from build123d import *

# Parameters (mm, degrees)
BOSS_EXTRUDE1_DEPTH = 3.03
BOSS_EXTRUDE2_DEPTH = 1
SKETCH3_W           = 1.3
SKETCH3_H           = 3
SKETCH3_W_2         = 1.5
SKETCH3_H_2         = 1.3
BOSS_EXTRUDE3_DEPTH = 5
BOSS_EXTRUDE4_DEPTH = 3
BOSS_EXTRUDE5_DEPTH = 1.5
SKETCH9_W           = 0.5
SKETCH9_H           = 2.5
BOSS_EXTRUDE6_DEPTH = 2
CUT_EXTRUDE1_DEPTH  = 0.5
SKETCH11_W          = 0.25
SKETCH11_H          = 2.5
BOSS_EXTRUDE7_DEPTH = 2
CUT_EXTRUDE2_DEPTH  = 0.25


with BuildPart() as part:
    # Sketch1 → Boss-Extrude1 (new body)
    with BuildSketch(Plane(origin=(0, 0, 0), x_dir=(1, 0, 0), z_dir=(0, 1, 0))):
        with BuildLine():
            Line((-16.7, -3.7), (16.7, -3.7))
            ThreePointArc((16.7, -3.7), (17.407106781, -3.407106781), (17.7, -2.7))
            Line((17.7, -2.7), (17.7, 2.7))
            ThreePointArc((17.7, 2.7), (17.407106781, 3.407106781), (16.7, 3.7))
            Line((16.7, 3.7), (-16.7, 3.7))
            ThreePointArc((-16.7, 3.7), (-17.407106781, 3.407106781), (-17.7, 2.7))
            Line((-17.7, 2.7), (-17.7, -2.7))
            ThreePointArc((-17.7, -2.7), (-17.407106781, -3.407106781), (-16.7, -3.7))
        make_face()
    extrude(amount=BOSS_EXTRUDE1_DEPTH)

    # Sketch2 → Boss-Extrude2 (add)
    with BuildSketch(Plane.XZ):
        with BuildLine():
            Line((16.7, 5.2), (-16.7, 5.2))
            ThreePointArc((-16.7, 5.2), (-18.467766953, 4.467766953), (-19.2, 2.7))
            Line((-19.2, 2.7), (-19.2, -2.7))
            ThreePointArc((-19.2, -2.7), (-18.467766953, -4.467766953), (-16.7, -5.2))
            Line((-16.7, -5.2), (16.7, -5.2))
            ThreePointArc((16.7, -5.2), (18.467766953, -4.467766953), (19.2, -2.7))
            Line((19.2, -2.7), (19.2, 2.7))
            ThreePointArc((19.2, 2.7), (18.467766953, 4.467766953), (16.7, 5.2))
        make_face()
    extrude(amount=-BOSS_EXTRUDE2_DEPTH)

    # Sketch3 → Boss-Extrude3 (add)
    with BuildSketch(Plane(origin=(0, 3.03, 0), x_dir=(1, 0, 0), z_dir=(0, 1, 0))):
        with Locations((-17.05, 0)):
            Rectangle(SKETCH3_W, SKETCH3_H)
        with Locations((-0.75, 3.05)):
            Rectangle(SKETCH3_W_2, SKETCH3_H_2)
    boss_extrude3 = extrude(amount=BOSS_EXTRUDE3_DEPTH)

    # Sketch5 → Boss-Extrude4 (add)
    with BuildSketch(Plane.XY.offset(1.5)):
        Polygon((-17.7, 8.03), (-18.733327763, 6.03), (-17.7, 6.03), align=None)
    boss_extrude4 = extrude(amount=-BOSS_EXTRUDE4_DEPTH)

    # Sketch8 → Boss-Extrude5 (add)
    with BuildSketch(Plane.ZY.offset(1.5)):
        Polygon((-3.7, 8.03), (-4.910348547, 6.03), (-3.7, 6.03), align=None)
    boss_extrude5 = extrude(amount=-BOSS_EXTRUDE5_DEPTH)

    # Sketch9 → Boss-Extrude6 (add)
    with BuildSketch(Plane(origin=(-16.4, 0, 0), x_dir=(0, 0, -1), z_dir=(1, 0, 0))):
        with Locations((0, 4.28)):
            Rectangle(SKETCH9_W, SKETCH9_H)
    boss_extrude6 = extrude(amount=BOSS_EXTRUDE6_DEPTH)

    # Sketch10 → Cut-Extrude1 (cut)
    with BuildSketch(Plane.XY.offset(0.25)):
        Polygon((-16.4, 5.53), (-14.4, 3.03), (-14.4, 5.53), align=None)
    cut_extrude1 = extrude(amount=-CUT_EXTRUDE1_DEPTH, mode=Mode.SUBTRACT)

    # Sketch11 → Boss-Extrude7 (add)
    with BuildSketch(Plane.XY.offset(-2.4)):
        with Locations((-0.125, 4.28)):
            Rectangle(SKETCH11_W, SKETCH11_H)
    boss_extrude7 = extrude(amount=BOSS_EXTRUDE7_DEPTH)

    # Sketch12 → Cut-Extrude2 (cut)
    with BuildSketch(Plane.ZY.offset(0.25)):
        Polygon((-2.4, 5.53), (-0.4, 3.03), (-0.4, 5.53), align=None)
    cut_extrude2 = extrude(amount=-CUT_EXTRUDE2_DEPTH, mode=Mode.SUBTRACT)

    # Mirror1: Boss-Extrude3, Boss-Extrude4, Boss-Extrude5, Boss-Extrude6, Cut-Extrude1, Boss-Extrude7, Cut-Extrude2 across plane
    add(boss_extrude3.mirror(Plane(origin=(0, 0, 0), x_dir=(0, 0, 1), z_dir=(1, 0, 0))))
    add(boss_extrude4.mirror(Plane(origin=(0, 0, 0), x_dir=(0, 0, 1), z_dir=(1, 0, 0))))
    add(boss_extrude5.mirror(Plane(origin=(0, 0, 0), x_dir=(0, 0, 1), z_dir=(1, 0, 0))))
    add(boss_extrude6.mirror(Plane(origin=(0, 0, 0), x_dir=(0, 0, 1), z_dir=(1, 0, 0))))
    add(cut_extrude1.mirror(Plane(origin=(0, 0, 0), x_dir=(0, 0, 1), z_dir=(1, 0, 0))), mode=Mode.SUBTRACT)
    add(boss_extrude7.mirror(Plane(origin=(0, 0, 0), x_dir=(0, 0, 1), z_dir=(1, 0, 0))))
    add(cut_extrude2.mirror(Plane(origin=(0, 0, 0), x_dir=(0, 0, 1), z_dir=(1, 0, 0))), mode=Mode.SUBTRACT)


solid = part.part
Work out the finished part from the listing and answer in its coordinate system (mm). A direction names the side the tool comes from. Round coordinates to 2 decimals unless told otherwise and drop trailing zeros. Order: outer loops, then holes, each group sorted by start corner. A loop starts at its lowest first (then second) coordinate and runs counter-clockwise, first axis right, second up. Notation, with made-up numbers: M 40,-39 L 76,-39 A6 cw 76,-30 Z; hole C -30,-10 d8. An arc over 180 degrees is marked long. Put each result on its own line as item: value. Start each with the question number.
Q1. Straight lines are drawn through the part: L1, parallel to Y at x = 15.5, z = -3; L2, parallel to Y at x = -14, z = -4.25; L3, parallel to Z at x = 13.5, y = 2.25. For each, find the intervals that lie inside material, in ascending order. Write a range as [from, to].
Q2. Section D-D, the plane y = 2.5 is taken. Write down the section's boundary in (x, z).
Q3. Section A-A, the plane y = 6.75 is taken. Write down the section's boundary in (x, z).
Q4. Section C-C, the plane x = -15 is taken. Write down the section's boundary in (y, z).
Q5. A tool of negligible diameter and unlimited length cuts with its end or side. For faces 1 (the cylindrical face through (17.399, 2.001, 3.415)), 2 (the flat face through (0.004, 4.297, -1.414)), 3 (the flat face through (-17, 6, -1.5)), 4 (the flat face through (16.4, 5.5, 0.4)), 5 (the cylindrical face through (-17.415, 2.001, 3.399)), from which of +Z, -Z, +X, -X, +Y, -Y can it reach the whole face along a straight path? Write none if from no direction.
Q6. Section B-B, the plane z = 1 is taken. Write down the section's boundary in (x, y).
Q7. For a pull along X with two mould halves and no side action, classify faces 6 (the cylindrical face through (-18.487, 0.493, -4.448)), 7 (the flat face through (-16.4, 5.5, 0.4)), 8 (the flat face through (17.7, 3, 0)) as pulls with the +X half, pulls with the -X half, needs draft (parallel to the pull), parting line crosses it, or undercut.
Q8. Flat-ended cylindrical pins translate along their axes: pin 1 (2 mm diameter, centred on y = 5.5, z = -3.5, fed in from -X); pin 2 (3 mm diameter, centred on y = 6, z = -3.5, fed in from +X); pin 3 (2 mm diameter, centred on x = 15.5, y = 4.5, fed in from +Z). Find the tip coordinate at first contact, or state that the pin passes through.
Findings below:
1. L1: y = [0, 3.03]
1. L2: y = [0, 1]
1. L3: z = [-3.7, 3.7]
2. outline: M -17.7,-2.7 A1 ccw -16.7,-3.7 L 16.7,-3.7 A1 ccw 17.7,-2.7 L 17.7,2.7 A1 ccw 16.7,3.7 L -16.7,3.7 A1 ccw -17.7,2.7 Z
3. outline: M -18.36,-1.5 L -16.4,-1.5 L -16.4,1.5 L -18.36,1.5 Z; M -1.5,-4.47 L 1.5,-4.47 L 1.5,-2.4 L -1.5,-2.4 Z; M 16.4,-1.5 L 18.36,-1.5 L 18.36,1.5 L 16.4,1.5 Z
4. outline: M 0,-5.2 L 1,-5.2 L 1,-3.7 L 3.03,-3.7 L 3.03,-0.25 L 3.78,-0.25 L 3.78,0.25 L 3.03,0.25 L 3.03,3.7 L 1,3.7 L 1,5.2 L 0,5.2 Z
5. face 1: +Z, +X, +Y
5. face 2: +Z, +Y
5. face 3: -Z, -X, +Y
5. face 4: +Y
5. face 5: +Z, -X, +Y
6. outline: M -19.2,0 L 19.2,0 L 19.2,1 L 17.7,1 L 17.7,6.03 L 18.73,6.03 L 17.7,8.03 L 16.4,8.03 L 16.4,3.03 L -16.4,3.03 L -16.4,8.03 L -17.7,8.03 L -18.73,6.03 L -17.7,6.03 L -17.7,1 L -19.2,1 Z
7. face 6: pulls with the -X half
7. face 7: undercut
7. face 8: pulls with the +X half
8. pin 1: stops at x = -1.5
8. pin 2: stops at x = 1.5
8. pin 3: stops at z = 1.5
